Read the model definition and answer for the solid it produces. Units are mm, in the model's axes. Face numbers are marked on the shaded views. A direction names the side the tool comes from. Coordinates: 2 decimals unless noted, no trailing zeros. Order: outer loops, then holes, each group sorted by start corner. A loop starts at its lowest first (then second) coordinate and runs counter-clockwise, first axis right, second up. Notation, with made-up numbers: M -4,20.5 L 40,20.5 A22 cw 40,32.5 Z; hole C -28.5,14.25 d1. An arc over 180 degrees is marked long. Write each question's results on one line, items separated by ' | '.
```python
from build123d import *

# Parameters (mm, degrees)
MAIN_ANGLE          = 180
CIRCULAR_BOSS_REACH = 111.487
SKETCH6_R           = 11.1125
CIRCULAR_CUT_DEPTH  = 110.4866698
SKETCH7_W           = 4.7625
SKETCH7_H           = 3.175


with BuildPart() as part:
    # Sketch1 → Main (revolve)
    with BuildSketch(Plane(origin=(0, 0, 0), x_dir=(0, 0, -1), z_dir=(1, 0, 0))):
        Polygon((38.1, 88.9), (0, 88.9), (0, 84.1375), (28.575, 84.1375), (28.575, 44.45), (34.925, 44.45), (34.925, 4.7625), (33.3375, 4.7625), (33.3375, 0), (38.1, 0), align=None)
    revolve(axis=Axis((0, 88.9, 0), (0, 1, 0)), revolution_arc=MAIN_ANGLE)

    # Sketch5 → Circular Boss (add, up to next)
    with BuildSketch(Plane.XY.offset(13.208), mode=Mode.PRIVATE) as circular_boss_sk1:
        with BuildLine():
            Line((0, 30.1625), (0, 58.7375))
            ThreePointArc((0, 58.7375), (-14.2875, 44.45), (0, 30.1625))
        make_face()
    circular_boss_tool1 = extrude(circular_boss_sk1.sketch, amount=CIRCULAR_BOSS_REACH, mode=Mode.PRIVATE) - part.part
    add(circular_boss_tool1.solids().sort_by_distance((-6.063803, 44.45, 13.208))[0])

    # Sketch6 → Circular Cut (cut, through all)
    with BuildSketch(Plane.XY.offset(13.208)):
        with Locations((0, 44.45)):
            Circle(SKETCH6_R)
    extrude(amount=CIRCULAR_CUT_DEPTH, mode=Mode.SUBTRACT)

    # Sketch7 → Cut-Revolve1 (revolve, cut)
    with BuildSketch(Plane(origin=(0, 7.447290845, 55.242674731), x_dir=(0, 0, -1), z_dir=(1, 0, 0))):
        with Locations((90.961424731, 63.990209155)):
            Rectangle(SKETCH7_W, SKETCH7_H)
    revolve(axis=Axis((0, 73.025, 0), (0, -1, 0)), mode=Mode.SUBTRACT)


solid = part.part
```
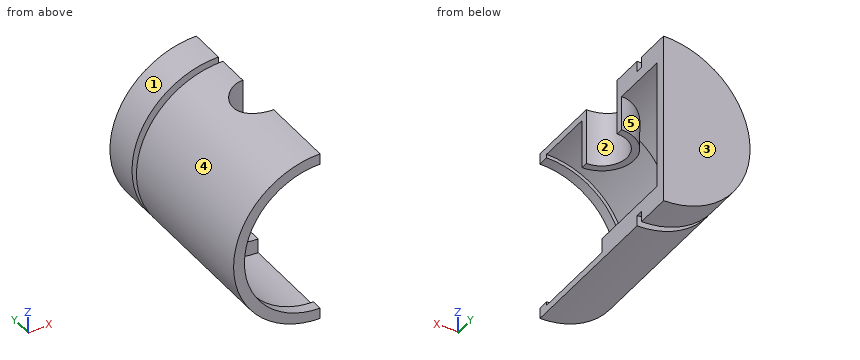
(1) For the marked faces 4 and 5, determine the directions among +Z, -Z, +X, -X, +Y, -Y from which every point of the face is accessible in a straight line to the end or side of a thin tool.
Conclusion:
face 4: -X, +Y, -Y | face 5: none
(2) Straight lines are drawn through the part: line 1 (Y direction, x = -23, z = -20); line 2 (Z direction, x = -7.5, y = 57); line 3 (Z direction, x = -22, y = 52). For each, find the intervals that lie inside material, in ascending order.
Conclusion:
line 1: 44.45 to 88.9 | line 2: -37.35 to -27.57, 27.57 to 37.35 | line 3: -31.11 to -18.24, 18.24 to 31.11
(3) The mould has two halves that part along Y. Classify the marked faces 1, 2 and 3: pulls with the +Y half, pulls with the -Y half, needs draft (parallel to the pull), parting line crosses it, or undercut.
Conclusion:
face 1: needs draft | face 2: undercut | face 3: pulls with the +Y half
(4) The part is cut by section C-C, the plane y = 40. Write down the section's boundary in (x, z) (3 decimals), then the cut area to 3 significant figures.
Conclusion:
outline: M -13.577,13.208 L -10.183,13.208 L -10.183,36.714 A38.1 ccw 0,-38.1 L 0,-34.925 A34.925 cw -13.577,32.178 Z | area: 398 mm²
(5) Given pin 1 (10.5 mm diameter, centred on x = -15.5, z = -6, fed in from -Y); pin 2 (10 mm diameter, centred on x = -27, y = 71.5, fed in from +Z); pin 3 (10 mm diameter, centred on x = -21, y = 62, fed in from -Z), each flat-ended and moving along its own axis, determine where each tip first touches the part or whether it passes through.
Conclusion:
pin 1: y = 84.14 | pin 2: z = 30.94 | pin 3: z = -34.58
